The drawing under review shows one solid part. Ordinate dimensions are in mm from its lowest x, y, z. Round coordinates to 2 decimals unless told otherwise and drop trailing zeros. Order: outer loops, then holes, each group sorted by start corner. A loop starts at its lowest first (then second) coordinate and runs counter-clockwise, first axis right, second up. Notation, with made-up numbers: M -13.75,11.5 L 32.25,11.5 A31 cw 32.25,50.5 Z; hole C 66,20 d8. An arc over 180 degrees is marked long. Write item = value, one per line. Start each with the question number.
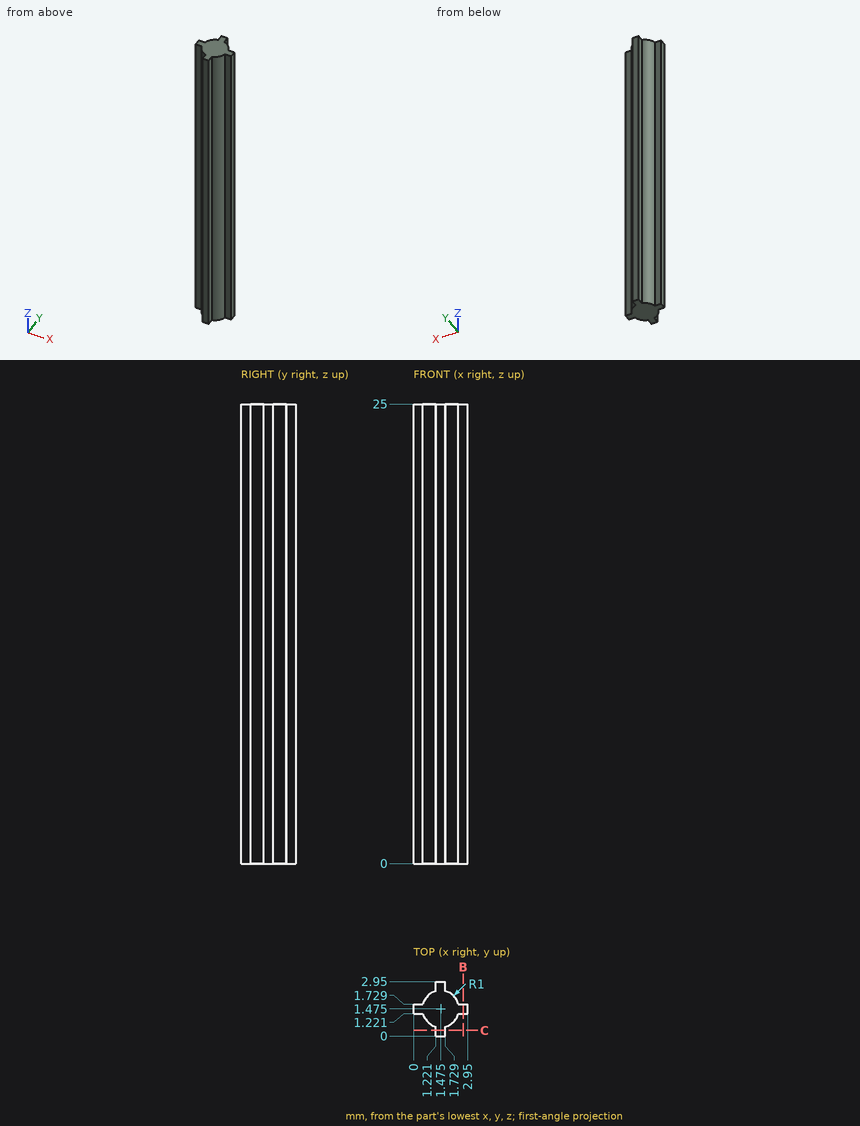
(1) For line 1 along X through (y, z) = (2.65, 12.25); line 2 along X through (y, z) = (2.2, 7.5) (1 decimal), list the stretches that pass through material, from the lowest coordinate up. Write a range as [from, to].
(2) Consider section B-B, the plane x = 2.7. Write out the cut boundary in (y, z).
(3) Insertion check: pin 1 (1.5 mm diameter, centred on x = 1.5, z = 10.5, fed in from -Y); pin 2 (1 mm diameter, centred on y = 0.5, z = 13.5, fed in from -X) (1 decimal); pin 3 (0.6 mm diameter, centred on y = 0.5, z = 12.5, fed in from +X); pin 4 (0.6 mm diameter, centred on x = 0, z = 7.5, fed in from -Y). Each pin has a flat end and moves straight along its axis. Give the tip position at first contact, or say it passes through.
Completed:
q1.line_1 = [1.22, 1.73]
q1.line_2 = [0.8, 2.2]
q2.outline = M 1.22,0 L 1.73,0 L 1.73,25 L 1.22,25 Z
q3.pin_1 = 0
q3.pin_2 = 0.6
q3.pin_3 = 2.21
q3.pin_4 = 1.22
